from build123d import *

# Parameters (mm, degrees)
F0_R     = 2.54
F1_DEPTH = 0.9525
F2_R     = 2.54
F3_DEPTH = 0.9398


with BuildPart() as f1:
    # F0 (on Front) → F1 (new body)
    with BuildSketch(Plane.XZ):
        with BuildLine():
            Line((39.6875, 0), (39.6875, 63.5))
            Line((39.6875, 63.5), (-39.6875, 63.5))
            Line((-39.6875, 63.5), (-39.6875, 0))
            Line((-39.6875, 0), (-33.02, 0))
            ThreePointArc((-33.02, 0), (-30.48, 2.54), (-27.94, 0))
            Line((-27.94, 0), (-17.78, 0))
            ThreePointArc((-17.78, 0), (-15.24, 2.54), (-12.7, 0))
            Line((-12.7, 0), (-2.54, 0))
            ThreePointArc((-2.54, 0), (0, 2.54), (2.54, 0))
            Line((2.54, 0), (12.7, 0))
            ThreePointArc((12.7, 0), (15.24, 2.54), (17.78, 0))
            Line((17.78, 0), (27.94, 0))
            ThreePointArc((27.94, 0), (30.48, 2.54), (33.02, 0))
            Line((33.02, 0), (39.6875, 0))
        make_face()
        with Locations((-30.48, 25.4)):
            Circle(F0_R, mode=Mode.SUBTRACT)
        with Locations((-15.24, 25.4)):
            Circle(F0_R, mode=Mode.SUBTRACT)
        with Locations((0, 25.4)):
            Circle(F0_R, mode=Mode.SUBTRACT)
        with Locations((15.24, 25.4)):
            Circle(F0_R, mode=Mode.SUBTRACT)
        with Locations((30.48, 25.4)):
            Circle(F0_R, mode=Mode.SUBTRACT)
        with Locations((-30.48, 50.8)):
            Circle(F0_R, mode=Mode.SUBTRACT)
        with Locations((-15.24, 50.8)):
            Circle(F0_R, mode=Mode.SUBTRACT)
        with Locations((0, 50.8)):
            Circle(F0_R, mode=Mode.SUBTRACT)
        with Locations((15.24, 50.8)):
            Circle(F0_R, mode=Mode.SUBTRACT)
    extrude(amount=-F1_DEPTH)

    # F2 (on Top) → F3 (join)
    with BuildSketch(Plane.XY):
        with BuildLine():
            Line((39.6875, 0), (39.6875, 63.5))
            Line((39.6875, 63.5), (-39.6875, 63.5))
            Line((-39.6875, 63.5), (-39.6875, 0))
            Line((-39.6875, 0), (-33.02, 0))
            ThreePointArc((-33.02, 0), (-30.48, 2.54), (-27.94, 0))
            Line((-27.94, 0), (-17.78, 0))
            ThreePointArc((-17.78, 0), (-15.24, 2.54), (-12.7, 0))
            Line((-12.7, 0), (-2.54, 0))
            ThreePointArc((-2.54, 0), (0, 2.54), (2.54, 0))
            Line((2.54, 0), (12.7, 0))
            ThreePointArc((12.7, 0), (15.24, 2.54), (17.78, 0))
            Line((17.78, 0), (27.94, 0))
            ThreePointArc((27.94, 0), (30.48, 2.54), (33.02, 0))
            Line((33.02, 0), (39.6875, 0))
        make_face()
        with Locations((-30.48, 25.4)):
            Circle(F2_R, mode=Mode.SUBTRACT)
        with Locations((-15.24, 25.4)):
            Circle(F2_R, mode=Mode.SUBTRACT)
        with Locations((0, 25.4)):
            Circle(F2_R, mode=Mode.SUBTRACT)
        with Locations((15.24, 25.4)):
            Circle(F2_R, mode=Mode.SUBTRACT)
        with Locations((30.48, 25.4)):
            Circle(F2_R, mode=Mode.SUBTRACT)
        with Locations((-30.48, 50.8)):
            Circle(F2_R, mode=Mode.SUBTRACT)
        with Locations((-15.24, 50.8)):
            Circle(F2_R, mode=Mode.SUBTRACT)
        with Locations((0, 50.8)):
            Circle(F2_R, mode=Mode.SUBTRACT)
        with Locations((15.24, 50.8)):
            Circle(F2_R, mode=Mode.SUBTRACT)
        with Locations((30.48, 50.8)):
            Circle(F2_R, mode=Mode.SUBTRACT)
    extrude(amount=-F3_DEPTH)


solid = f1.part
Work out the finished part from the listing and answer in its coordinate system (mm). A direction names the side the tool comes from. Give positions to 0.01 mm unless a question says otherwise; leave off trailing zeros. Write each loop counter-clockwise with the first axis right and the second up, starting at its lowest first coordinate (ties: lowest second). Pieces come first, ordered by that corner, then holes. Notation, with made-up numbers: (6, 26.25) - (27, 26.25) arc R23 cw to (27, 58.25) - close; hole circle Ø5 at (-15.75, 10.25). An arc over 180 degrees is marked (long way). One line per item, written item: value. Start each with the question number.
1. For faces 4 (the cylindrical face through (15.18, 2.54, -0.46)), 5 (the cylindrical face through (14.69, 0.47, 48.32)), determine the directions among +Z, -Z, +X, -X, +Y, -Y from which every point of the face is accessible in a straight line to the end or side of a thin tool.
2. Find section A-A (y = 50.8). Write down the section's boundary in (x, z), then the cut area to 3 significant figures.
3. For a pull along Y with two mould halves and no side action, classify faces 1 (the cylindrical face through (-0.33, 27.92, -0.46)), 2 (the cylindrical face through (30.42, 2.54, -0.46)), 3 (the cylindrical face through (-15.57, 0.47, 27.92)) as +Y half, -Y half, draft (parallel to the pull), parting line (faces both ways), or undercut.
4. Given pin 1 (1 mm diameter, centred on x = 4.5, z = 39.5, fed in from +Y); pin 2 (4.5 mm diameter, centred on x = 0, y = 50.8, fed in from +Z); pin 3 (6.5 mm diameter, centred on x = 0, y = 25.4, fed in from +Z), each flat-ended and moving along its own axis, determine where each tip first touches the part or whether it passes through.
5. Find section D-D (x = -22). Write down the section's boundary in (y, z), then the cut area to 3 significant figures.
6. Find section B-B (x = 0). Write down the section's boundary in (y, z), then the cut area to 3 significant figures.
7. Find section C-C (x = 30.48). Write down the section's boundary in (y, z), then the cut area to 3 significant figures.
8. Consider probe 1 along Y at (x, z) = (-15.24, -0.55); probe 2 along Y at (x, z) = (9.5, 3). Determine where each line is inside the solid, lowest interval first.
Geometry results:
1. face 4: -Z, -Y
1. face 5: +Y, -Y
2. outline: (-39.69, -0.94) - (-33.02, -0.94) - (-33.02, 0) - (-39.69, 0) - close; (-27.94, -0.94) - (-17.78, -0.94) - (-17.78, 0) - (-27.94, 0) - close; (-12.7, -0.94) - (-2.54, -0.94) - (-2.54, 0) - (-12.7, 0) - close; (2.54, -0.94) - (12.7, -0.94) - (12.7, 0) - (2.54, 0) - close; (17.78, -0.94) - (27.94, -0.94) - (27.94, 0) - (17.78, 0) - close; (33.02, -0.94) - (39.69, -0.94) - (39.69, 0) - (33.02, 0) - close
2. area: 50.7 mm2
3. face 1: undercut
3. face 2: -Y half
3. face 3: draft
4. pin 1: y = 0.95
4. pin 2: through
4. pin 3: z = 0
5. outline: (0, -0.94) - (63.5, -0.94) - (63.5, 0) - (0.95, 0) - (0.95, 63.5) - (0, 63.5) - close
5. area: 120 mm2
6. outline: (0, 2.54) - (0.95, 2.54) - (0.95, 22.86) - (0, 22.86) - close; (0, 27.94) - (0.95, 27.94) - (0.95, 48.26) - (0, 48.26) - close; (0, 53.34) - (0.95, 53.34) - (0.95, 63.5) - (0, 63.5) - close; (2.54, -0.94) - (22.86, -0.94) - (22.86, 0) - (2.54, 0) - close; (27.94, -0.94) - (48.26, -0.94) - (48.26, 0) - (27.94, 0) - close; (53.34, -0.94) - (63.5, -0.94) - (63.5, 0) - (53.34, 0) - close
6. area: 96.1 mm2
7. outline: (0, 2.54) - (0.95, 2.54) - (0.95, 22.86) - (0, 22.86) - close; (0, 27.94) - (0.95, 27.94) - (0.95, 63.5) - (0, 63.5) - close; (2.54, -0.94) - (22.86, -0.94) - (22.86, 0) - (2.54, 0) - close; (27.94, -0.94) - (48.26, -0.94) - (48.26, 0) - (27.94, 0) - close; (53.34, -0.94) - (63.5, -0.94) - (63.5, 0) - (53.34, 0) - close
7. area: 101 mm2
8. probe 1: 2.54 to 22.86, 27.94 to 48.26, 53.34 to 63.5
8. probe 2: 0 to 0.95
